```python
from build123d import *

# Parameters (mm, degrees)
SKETCH1_W           = 109
SKETCH1_H           = 12
BOSS_EXTRUDE1_DEPTH = 5
SKETCH2_R           = 5
CUT_EXTRUDE2_DEPTH  = 56.056788864
CUT_EXTRUDE3_DEPTH  = 56.056788864


with BuildPart() as part:
    # Sketch1 → Boss-Extrude1 (new body)
    with BuildSketch(Plane(origin=(0, 0, 0), x_dir=(1, 0, 0), z_dir=(0, 1, 0))):
        Rectangle(SKETCH1_W, SKETCH1_H)
    extrude(amount=BOSS_EXTRUDE1_DEPTH)

    # Sketch2 → Cut-Extrude2 (cut, through all)
    with BuildSketch(Plane(origin=(0, 5, 0), x_dir=(1, 0, 0), z_dir=(0, 1, 0))):
        with Locations(Location((0, 0, 0), (0, 0, 270))):
            Circle(SKETCH2_R)
    extrude(amount=-CUT_EXTRUDE2_DEPTH, mode=Mode.SUBTRACT)

    # Sketch3 → Cut-Extrude3 (cut, through all)
    with BuildSketch(Plane(origin=(0, 5, 0), x_dir=(1, 0, 0), z_dir=(0, 1, 0))):
        Polygon((-54.5, 0), (-54.5, 2.5), (-49.5, 2.5), (-49.5, -2.5), (-54.5, -2.5), align=None)
    cut_extrude3 = extrude(amount=-CUT_EXTRUDE3_DEPTH, mode=Mode.SUBTRACT)

    # Mirror1: Cut-Extrude3 across plane
    add(cut_extrude3.mirror(Plane(origin=(0, 0, 0), x_dir=(0, 0, 1), z_dir=(1, 0, 0))), mode=Mode.SUBTRACT)


solid = part.part
```
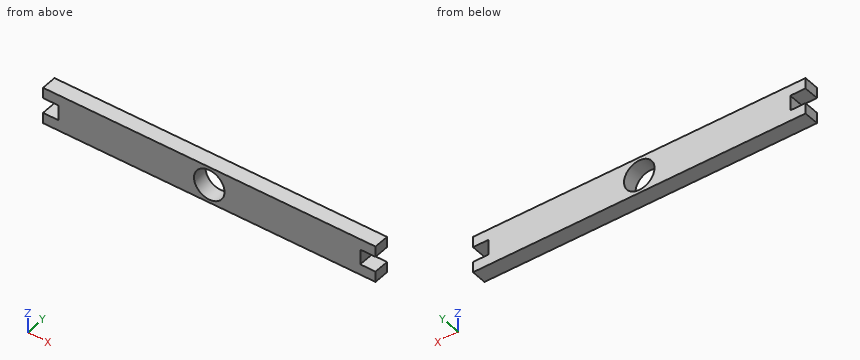
Read the model definition and answer for the solid it produces. Units are mm, in the model's axes. Give positions to 0.01 mm unless a question says otherwise; leave off trailing zeros. Loops run counter-clockwise (first coordinate to the right, second up) from the corner with the lowest first, then second, coordinate; pieces in that order, holes last.
Item 1: Each of these flat-tipped pins is pushed along its axis until it touches: pin 1 Ø1.5 at (y, z) = (2, -1) entering from +X; pin 2 Ø4 at (x, z) = (39, -0.5) entering from -Y. Where does it stop, or does it pass through?
Item 2: The part is cut by section C-C (y = 2.9). Write down the section's boundary in (x, z), and give its area (3 significant figures).
Item 3: The part is cut by section B-B (z = 0). Write down the section's boundary in (x, y).
Item 4: Find the intervals of material crossed by line 1 along X through (y, z) = (4.5, -0.25); line 2 along X through (y, z) = (4.7, 4.5), in increasing order.
Item 5: The part is cut by section A-A (x = 0). Write down the section's boundary in (y, z), and give its area (3 significant figures).
Taken from the geometry:
1. pin 1: stops at x = 49.5
1. pin 2: stops at y = 0
2. outline: (-54.5, -6) - (54.5, -6) - (54.5, -2.5) - (49.5, -2.5) - (49.5, 2.5) - (54.5, 2.5) - (54.5, 6) - (-54.5, 6) - (-54.5, 2.5) - (-49.5, 2.5) - (-49.5, -2.5) - (-54.5, -2.5) - close; hole circle Ø10 at (0, 0)
2. area: 1,180 mm2
3. outline: (-49.5, 0) - (-5, 0) - (-5, 5) - (-49.5, 5) - close; (5, 0) - (49.5, 0) - (49.5, 5) - (5, 5) - close
4. line 1: x = -49.5 to -4.99, 4.99 to 49.5
4. line 2: x = -54.5 to -2.18, 2.18 to 54.5
5. outline: (0, -6) - (5, -6) - (5, -5) - (0, -5) - close; (0, 5) - (5, 5) - (5, 6) - (0, 6) - close
5. area: 10.0 mm2
